from build123d import *

# Parameters (mm, degrees)
F1_DEPTH = 25.4


with BuildPart() as f1:
    # F0 (on Front) → F1 (new body)
    with BuildSketch(Plane.XZ):
        Polygon((12.860392, 0), (0, 35.152197), (-15.112189, 0), (-24.446175, -21.711619), (-39.281469, -56.219734), (0, -27.512548), (33.428319, -56.219734), (20.803563, -21.711619), align=None)
        Polygon((41.081976, 0), (12.860392, 0), (20.803563, -21.711619), align=None)
        Polygon((-24.446175, -21.711619), (-15.112189, 0), (-46.456773, 0), align=None)
    extrude(amount=F1_DEPTH)


solid = f1.part
Work out the finished part from the listing and answer in its coordinate system (mm). A direction names the side the tool comes from. Round coordinates to 2 decimals unless told otherwise and drop trailing zeros. Write each loop counter-clockwise with the first axis right and the second up, starting at its lowest first coordinate (ties: lowest second). Pieces come first, ordered by that corner, then holes.
1) A tool of negligible diameter and unlimited length cuts with its end or side. For faces 4 (the flat face through (-31, -13, 0)), 5 (the flat face through (-19.92, -12.52, -42.07)), 6 (the flat face through (27, -13, 0)), from which of +Z, -Z, +X, -X, +Y, -Y can it reach the whole face along a straight path? Write none if from no direction.
2) Straight lines are drawn through the part: line 1 (X direction, y = -8, z = -49.5); line 2 (Z direction, x = -27.5, y = -14.5); line 3 (X direction, y = -3, z = -31). For each, find the intervals that lie inside material, in ascending order.
3) A cutting plane is placed at C-C (y = -4.5). Give the vertices of the cut face in (x, z), plus the area to 3 significant figures.
4) A cutting plane is placed at D-D (z = 6.5). Give the vertices of the cut face in (x, y).
5) The mould has two halves that part along X. Classify faces 1 (the flat face through (-3, -25.4, -14)), 2 (the flat face through (-31.76, -12.52, -38.72)), 3 (the flat face through (16.48, -12.522, -41.665)): pulls with the +X half, pulls with the -X half, needs draft (parallel to the pull), parting line crosses it, or undercut.
6) A cutting plane is placed at B-B (x = -37.5). Give the vertices of the cut face in (y, z).
7) Given pin 1 Ø1 at (x, y) = (-32, -15.5) entering from -Z; pin 2 Ø5 at (y, z) = (-4.5, 8.5) entering from +X; pin 3 Ø10 at (x, y) = (-17.5, -19.5) entering from +Z, each flat-ended and moving along its own axis, determine where each tip first touches the part or whether it passes through.
8) A cutting plane is placed at A-A (z = -40). Give the vertices of the cut face in (x, y).
Completed:
1. face 4: +Z, -X, +Y, -Y
1. face 5: -Z, +Y, -Y
1. face 6: +Z, +X, +Y, -Y
2. line 1: x = -36.39 to -30.09, 25.6 to 30.97
2. line 2: z = -47.61 to -28.82, -18.7 to 0
2. line 3: x = -28.44 to -4.77, 4.06 to 24.2
3. outline: (-46.46, 0) - (-24.45, -21.71) - (-39.28, -56.22) - (0, -27.51) - (33.43, -56.22) - (20.8, -21.71) - (41.08, 0) - (12.86, 0) - (0, 35.15) - (-15.11, 0) - close
3. area: 2,920 mm2
4. outline: (-12.32, -25.4) - (10.48, -25.4) - (10.48, 0) - (-12.32, 0) - close
5. face 1: needs draft
5. face 2: pulls with the -X half
5. face 3: undercut
6. outline: (-25.4, -54.92) - (0, -54.92) - (0, -52.08) - (-25.4, -52.08) - close; (-25.4, -8.84) - (0, -8.84) - (0, 0) - (-25.4, 0) - close
7. pin 1: stops at z = -51.26
7. pin 2: stops at x = 10.67
7. pin 3: stops at z = 6.08
8. outline: (-32.31, -25.4) - (-17.09, -25.4) - (-17.09, 0) - (-32.31, 0) - close; (14.54, -25.4) - (27.49, -25.4) - (27.49, 0) - (14.54, 0) - close
